Geometry: final body of the model. Coordinates: model frame, mm. Face numbers are marked on the shaded views. A direction names the side the tool comes from. Coordinates: 2 decimals unless noted, no trailing zeros. Write each loop counter-clockwise with the first axis right and the second up, starting at its lowest first coordinate (ties: lowest second). Pieces come first, ordered by that corner, then holes.
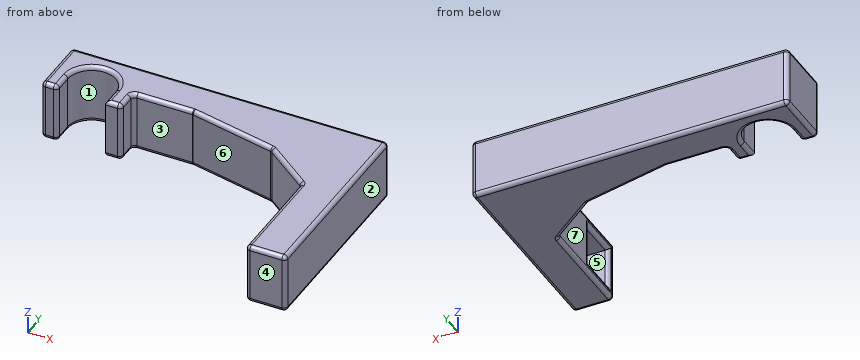
from build123d import *

# Parameters (mm, degrees)
F1_DEPTH = 30
F2_W     = 20.25
F2_H     = 20.25
F3_DEPTH = 15
F4_R     = 2


# Not quite as in the source:
# - a feature names something its author has since deleted; it is built from what else it names


with BuildPart() as f1:
    # F0 (on Top) → F1 (new body)
    with BuildSketch(Plane.XY):
        Polygon((-12, -5), (-12, 5), (-12, 25), (-20, 25), (-20, -5), align=None)
        with BuildLine():
            ThreePointArc((-12, 5), (0, 17), (12, 5))
            Line((12, 5), (12, 25))
            Line((12, 25), (-12, 25))
            Line((-12, 25), (-12, 5))
        make_face()
        Polygon((12, 25), (12, 5), (12, -5), (20, -5), (20, 6), (50, 6), (94.016642033, -3.3560260868), (118, -21.3781941203), (118, -75), (138, -75), (138, -15), (138, 25), align=None)
    extrude(amount=F1_DEPTH)

    # F2 (on face) → F3 (cut)
    with BuildSketch(Plane(origin=(118, 0, 0), x_dir=(0, -1, 0), z_dir=(-1, 0, 0))):
        with Locations((60, 15)):
            Rectangle(F2_W, F2_H)
    extrude(amount=-F3_DEPTH, mode=Mode.SUBTRACT)

    # F4
    f4_edges = [f1.edges().sort_by_distance(p)[0] for p in [
        (20, -5, 15),
        (20, 6, 15),
        (20, 0.5, 0),
        (20, 0.5, 30),
        (50, 6, 15),
        (35, 6, 0),
        (35, 6, 30),
        (94.016642, -3.356026, 15),
        (118, -21.378194, 15),
        (106.008321, -12.36711, 0),
        (106.008321, -12.36711, 30),
        (118, -48.189097, 0),
        (118, -48.189097, 30),
        (118, -75, 15),
        (118, -60, 4.875),
        (118, -49.875, 15),
        (118, -60, 25.125),
        (118, -70.125, 15),
        (138, -75, 15),
        (128, -75, 0),
        (128, -75, 30),
        (-20, 10, 30),
        (-16, -5, 30),
        (-12, 0, 30),
        (0, 17, 30),
        (12, 0, 30),
        (16, -5, 30),
        (72.008321, 1.321987, 30),
        (138, -25, 30),
        (59, 25, 30),
        (-20, 10, 0),
        (-16, -5, 0),
        (-12, 0, 0),
        (0, 17, 0),
        (12, 0, 0),
        (16, -5, 0),
        (72.008321, 1.321987, 0),
        (138, -25, 0),
        (59, 25, 0),
        (-20, -5, 15),
        (-12, -5, 15),
        (138, 25, 15),
        (-20, 25, 15),
    ]]
    fillet(f4_edges, radius=F4_R)


solid = f1.part
Item 1: Pin query (flat end, axial travel): pin 1 (2 mm diameter, centred on x = 62, z = 6.5, fed in from -Y); pin 2 (6 mm diameter, centred on x = 35.5, y = 5, fed in from +Z); pin 3 (1 mm diameter, centred on x = 5, z = 11, fed in from -Y); pin 4 (5 mm diameter, centred on y = -6.5, z = 21, fed in from -X). Return the tip coordinate at first contact, or that it passes through.
Derived:
pin 1: stops at y = 3.24
pin 2: stops at z = 30
pin 3: stops at y = 15.67
pin 4: stops at x = -19.73
Item 2: Pull-direction query (X, two-part tool) for the marked faces 1, 2, 3 and 4; classes: released by +X, released by -X, zero draft, split by the parting line, or undercut.
Derived:
face 1: undercut
face 2: released by +X
face 3: undercut
face 4: zero draft
Item 3: Section B-B, the plane x = 0. Output: boundary loops of the cut face in (y, z), plus the area to 3 significant figures.
Derived:
outline: (17, 2) arc R2 ccw to (19, 0) - (23, 0) arc R2 ccw to (25, 2) - (25, 28) arc R2 ccw to (23, 30) - (19, 30) arc R2 ccw to (17, 28) - close
area: 237 mm2
Item 4: Material intervals for probe 1 along Y at (x, z) = (24.5, 22.5); probe 2 along Y at (x, z) = (-14, 23); probe 3 along X at (y, z) = (7, 7), sorted ascending.
Derived:
probe 1: y = 6 to 25
probe 2: y = -5 to 25
probe 3: x = -20 to -11.83, 11.83 to 138
Item 5: Set-up query: the marked faces 5, 6 and 7. Return all of +Z, -Z, +X, -X, +Y, -Y with unobstructed straight access to the full face (end or side cutting, diameter ignored); none if empty.
Derived:
face 5: -X
face 6: +Z, -Z, -Y
face 7: +Z, -Z, -X, -Y
Item 6: Section A-A, the plane y = -32. Output: boundary loops of the cut face in (x, z).
Derived:
outline: (118, 2) arc R2 ccw to (120, 0) - (136, 0) arc R2 ccw to (138, 2) - (138, 28) arc R2 ccw to (136, 30) - (120, 30) arc R2 ccw to (118, 28) - close
Item 7: Section D-D, the plane y = -52.5. Output: boundary loops of the cut face in (x, z) (3 decimals), plus the area to 3 significant figures.
Derived:
outline: (118, 2) arc R2 ccw to (120, 0) - (136, 0) arc R2 ccw to (138, 2) - (138, 28) arc R2 ccw to (136, 30) - (120, 30) arc R2 ccw to (118, 28) - (118, 27.125) arc R2 ccw to (120, 25.125) - (133, 25.125) - (133, 4.875) - (120, 4.875) arc R2 ccw to (118, 2.875) - close
area: 291 mm2
